from build123d import *

# Parameters (mm, degrees)
F0_R     = 17.145
F0_R_2   = 15.875
F1_DEPTH = 25.4
F2_R     = 17.145
F3_DEPTH = 5.08
F4_R     = 4.191
F5_DEPTH = 5.08


# Not quite as in the source:
# - after a boolean that leaves OpenCascade's solid faulty, fix() repairs it


with BuildPart() as f1:
    # F0 (on Front) → F1 (new body)
    with BuildSketch(Plane.XZ):
        Circle(F0_R)
        Circle(F0_R_2, mode=Mode.SUBTRACT)
    extrude(amount=F1_DEPTH)

    # F2 (on face) → F3 (join)
    with BuildSketch(Plane(origin=(0, 0, 0), x_dir=(-1, 0, 0), z_dir=(0, 1, 0))):
        Circle(F2_R)
    extrude(amount=F3_DEPTH)

    # F4 (on face) → F5 (join, through all)
    with BuildSketch(Plane.XZ):
        with BuildLine():
            add(Edge.make_bspline(
                [(9.525, 93.218), (9.3322422676, 59.4415284404), (17.145, 33.7770215762), (17.145, 0)],
                knots=[0, 0, 0, 0, 93.5289256006, 93.5289256006, 93.5289256006, 93.5289256006], degree=3))
            ThreePointArc((9.525, 93.218), (15.4919111989, 107.486755876), (1.1437665087, 101.7133541532))
            Line((1.1437665087, 101.7133541532), (0, 17.145))
            ThreePointArc((0, 17.145), (12.1233457634, 12.1233457634), (17.145, 0))
        make_face()
        with Locations((9.525, 101.6)):
            Circle(F4_R, mode=Mode.SUBTRACT)
        with BuildLine():
            ThreePointArc((-17.1425003406, 0.2927577006), (-12.0193946233, 12.2264131244), (0, 17.145))
            Line((0, 17.145), (-1.1437665087, 101.7133541532))
            ThreePointArc((-1.1437665087, 101.7133541532), (-15.4919111989, 107.486755876), (-9.525, 93.218))
            add(Edge.make_bspline(
                [(-9.525, 93.218), (-10.0234570054, 59.5641158888), (-16.5685631435, 33.8997937459), (-17.1425003406, 0.2927577006)],
                knots=[0, 0, 0, 0, 93.2585047549, 93.2585047549, 93.2585047549, 93.2585047549], degree=3))
        make_face()
        with Locations((-9.525, 101.6)):
            Circle(F4_R, mode=Mode.SUBTRACT)
    extrude(amount=-F5_DEPTH)

    add(f1.part.fix(), mode=Mode.REPLACE)


solid = f1.part
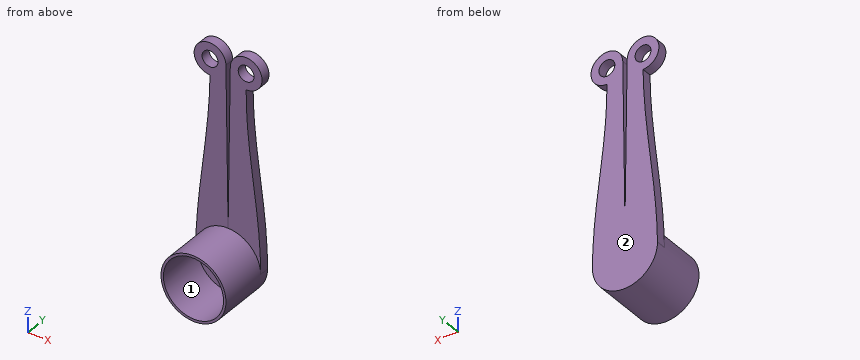
The listing builds one solid part. Answer for the finished solid, in the listing's coordinates (mm). Face numbers are marked on the shaded views. Round coordinates to 2 decimals unless told otherwise and drop trailing zeros. Write each loop counter-clockwise with the first axis right and the second up, starting at its lowest first coordinate (ties: lowest second). Pieces come first, ordered by that corner, then holes. Notation, with made-up numbers: M 62,76.5 L 115,76.5 A28 cw 115,100.5 Z; hole C 46,-8 d5. An arc over 180 degrees is marked long. Write each question's results on one line, items separated by ' | '. Start each with the question number.
Item 1: Given pin 1 Ø7.5 at (x, z) = (9.525, 101.6) entering from -Y; pin 2 Ø4 at (x, z) = (-0.5, 60.5) entering from +Y; pin 3 Ø8 at (y, z) = (-3, 36.5) entering from -X; pin 4 Ø12 at (x, y) = (-7.5, -22) entering from +Z, each flat-ended and moving along its own axis, determine where each tip first touches the part or whether it passes through.
Item 2: Find section B-B on x = 2.5. Write down the section's boundary in (y, z).
Item 3: Find section A-A on y = -19. Write down the section's boundary in (x, z) (3 decimals), and give its area (3 significant figures).
Item 4: Find section C-C on x = -12.5. Give the number of separate pieces and of enclosed holes in the cut face, and give its area (3 significant figures).
Item 5: Straight lines are drawn through the part: probe 1 along X at (y, z) = (-22, 0.5); probe 2 along Z at (x, y) = (0, -10) (3 decimals); probe 3 along Y at (x, z) = (5, 22.5). For each, find the intervals that lie inside material, in ascending order.
Item 6: The mould has two halves that part along Z. Classify the marked faces 1 and 2: +Z half, -Z half, draft (parallel to the pull), parting line (faces both ways), or undercut.
Answer block:
1) pin 1: passes through | pin 2: stops at y = 5.08 | pin 3: stops at x = -14.8 | pin 4: stops at z = 17.08
2) outline: M -25.4,-16.96 L 5.08,-16.96 L 5.08,106.17 L 0,106.17 L 0,16.96 L -25.4,16.96 L -25.4,15.68 L 0,15.68 L 0,-15.68 L -25.4,-15.68 Z
3) outline: C 0,0 d34.29; hole C 0,0 d31.75 | area: 132 mm²
4) separate pieces: 3 | enclosed holes: 0 | area: 480 mm²
5) probe 1: x = -17.14 to -15.87, 15.87 to 17.14 | probe 2: z = -17.145 to -15.875, 15.875 to 17.145 | probe 3: y = 0 to 5.08
6) face 1: undercut | face 2: draft
